Check sheet for the modelled part. Datum: model origin and axes. Units: mm. Face numbers are marked on the shaded views. A direction names the side the tool comes from. Coordinates: 2 decimals unless noted, no trailing zeros. Write each loop counter-clockwise with the first axis right and the second up, starting at its lowest first coordinate (ties: lowest second). Pieces come first, ordered by that corner, then holes. Notation, with made-up numbers: (12.25, 49.25) - (28.25, 49.25) arc R27 cw to (28.25, 70.25) - close; hole circle Ø4 at (-0.5, 62). An arc over 180 degrees is marked (long way). Write each question's results on one line, items separated by ' | '.
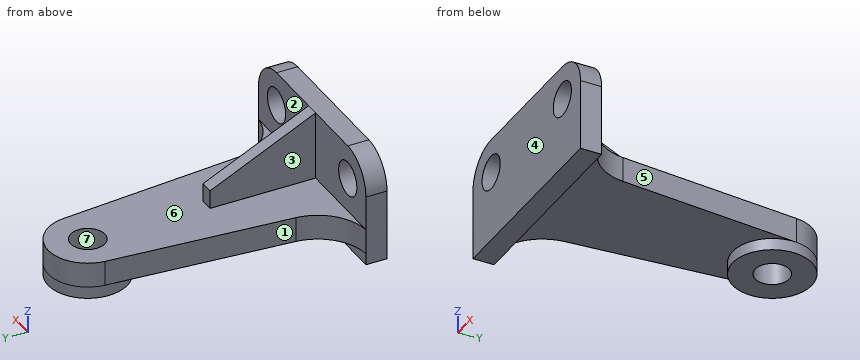
from build123d import *

# Parameters (mm, degrees)
EXTRUDE_1_DEPTH     = 8
SKETCH_2_R          = 6.5
CUT_EXTRUDE_1_DEPTH = 8
EXTRUDE_2_DEPTH     = 9.5
SKETCH_4_R          = 15
EXTRUDE_3_DEPTH     = 4.5
SKETCH_5_R          = 6.5
CUT_EXTRUDE_2_DEPTH = 41
EXTRUDE_4_DEPTH     = 2.5


with BuildPart() as part:
    # 스케치1 → 보스-돌출1 (new body)
    with BuildSketch(Plane(origin=(0, 0, 0), x_dir=(1, 0, 0), z_dir=(0, 1, 0))):
        with BuildLine():
            Line((-38.5, 40), (38.5, 40))
            Line((38.5, 40), (38.5, 13))
            ThreePointArc((38.5, 13), (34.692388155, 3.807611845), (25.5, 0))
            Line((25.5, 0), (-25.5, 0))
            ThreePointArc((-25.5, 0), (-34.692388155, 3.807611845), (-38.5, 13))
            Line((-38.5, 13), (-38.5, 40))
        make_face()
    extrude(amount=EXTRUDE_1_DEPTH)

    # 스케치2 → 컷-돌출1 (cut)
    with BuildSketch(Plane(origin=(0, 8, 0), x_dir=(1, 0, 0), z_dir=(0, 1, 0))):
        with Locations((-25.5, 13)):
            Circle(SKETCH_2_R)
        with Locations((25.5, 13)):
            Circle(SKETCH_2_R)
    extrude(amount=-CUT_EXTRUDE_1_DEPTH, mode=Mode.SUBTRACT)

    # 스케치3 → 보스-돌출2 (add)
    with BuildSketch(Plane(origin=(0, 0, -26), x_dir=(-1, 0, 0), z_dir=(0, 0, -1))):
        with BuildLine():
            Line((-38.5, 0), (-38.5, 8))
            ThreePointArc((-38.5, 8), (-26.561663341, 13.425258865), (-20.981002143, 25.291746827))
            Line((-20.981002143, 25.291746827), (-14.942920471, 94.307336141))
            ThreePointArc((-14.942920471, 94.307336141), (0, 108), (14.942920471, 94.307336141))
            Line((14.942920471, 94.307336141), (20.981002143, 25.291746827))
            ThreePointArc((20.981002143, 25.291746827), (26.561663341, 13.425258865), (38.5, 8))
            Line((38.5, 8), (38.5, 0))
            Line((38.5, 0), (-38.5, 0))
        make_face()
    extrude(amount=EXTRUDE_2_DEPTH)

    # 스케치4 → 보스-돌출3 (add)
    with BuildSketch(Plane(origin=(0, 0, -35.5), x_dir=(-1, 0, 0), z_dir=(0, 0, -1))):
        with Locations((0, 93)):
            Circle(SKETCH_4_R)
    extrude(amount=EXTRUDE_3_DEPTH)

    # 스케치5 → 컷-돌출2 (cut, through all)
    with BuildSketch(Plane(origin=(0, 0, -40), x_dir=(-1, 0, 0), z_dir=(0, 0, -1))):
        with Locations((0, 93)):
            Circle(SKETCH_5_R)
    extrude(amount=-CUT_EXTRUDE_2_DEPTH, mode=Mode.SUBTRACT)

    # 스케치7 → 보스-돌출4 (add, symmetric)
    with BuildSketch(Plane(origin=(0, 0, 0), x_dir=(0, 0, -1), z_dir=(1, 0, 0))):
        Polygon((0, 8), (35.5, 8), (35.5, 48), (19, 48), align=None)
    extrude(amount=EXTRUDE_4_DEPTH, both=True)


solid = part.part
1. Material ranges on L1, parallel to X at y = 3.25, z = -13; L2, parallel to Y at x = 0, z = -35.25; L3, parallel to Z at x = 25, y = 3, recorded low to high. Write a range as [from, to].
Values follow:
L1: x = [-38.5, -32], [-19, 19], [32, 38.5] | L2: y = [0, 86.5], [99.5, 108] | L3: z = [-40, -19.48], [-6.52, 0]
2. Sectioned sample at A-A (z = -28). Record the cut outline in (x, y), then the cut area to 3 significant figures.
Values follow:
outline: (-38.5, 0) - (38.5, 0) - (38.5, 8) arc R19 cw to (20.98, 25.29) - (14.94, 94.31) arc R15 ccw to (-14.94, 94.31) - (-20.98, 25.29) arc R19 cw to (-38.5, 8) - close; hole circle Ø13 at (0, 93) | area: 4,150 mm^2
3. Sectioned sample at C-C (z = -9). Record the cut outline in (x, y).
Values follow:
outline: (-37.87, 0) - (-30.62, 0) - (-30.62, 8) - (-37.87, 8) - close; (-20.38, 0) - (20.38, 0) - (20.38, 8) - (2.5, 8) - (2.5, 26.95) - (-2.5, 26.95) - (-2.5, 8) - (-20.38, 8) - close; (30.62, 0) - (37.87, 0) - (37.87, 8) - (30.62, 8) - close
4. Go/stop test with flat-tipped pins: pin 1 (1 mm diameter, centred on y = 42, z = -19.5, fed in from -X); pin 2 (21 mm diameter, centred on x = -25.5, z = -13, fed in from -Y); pin 3 (6 mm diameter, centred on x = -9.5, y = 46, fed in from +Z); pin 4 (23 mm diameter, centred on x = 15, y = 61.5, fed in from -Z). Record where each tip stops, or that it passes through.
Values follow:
pin 1: stops at x = -2.5 | pin 2: stops at y = 0 | pin 3: stops at z = -26 | pin 4: stops at z = -35.5
5. Access from +Z, -Z, +X, -X, +Y, -Y to the whole of each face (thin tool, end or side, straight path). Record for the marked faces 1, 2 and 3.
Values follow:
face 1: +Z, -Z, -X, +Y | face 2: +Z, +X, +Y | face 3: +Z, -X, +Y
6. Draft check along Y on the marked faces 4, 5, 6 and 7. Enter one of: pulls with the +Y half, pulls with the -Y half, needs draft (parallel to the pull), parting line crosses it, or undercut.
Values follow:
face 4: pulls with the -Y half | face 5: pulls with the +Y half | face 6: needs draft | face 7: undercut
7. Sectioned sample at B-B (x = -29). Record the cut outline in (y, z), then the cut area to 3 significant figures.
Values follow:
outline: (0, -40) - (8, -40) - (8, -35.5) - (11.39, -35.5) - (11.39, -26) - (8, -26) - (8, -18.48) - (0, -18.48) - close; (0, -7.52) - (8, -7.52) - (8, -0.48) - (0, -0.48) - close | area: 261 mm^2
8. Sectioned sample at D-D (y = 93). Record the cut outline in (x, z), then the cut area to 3 significant figures.
Values follow:
outline: (-15.06, -35.5) - (-15, -35.5) - (-15, -40) - (-6.5, -40) - (-6.5, -26) - (-15.06, -26) - close; (6.5, -40) - (15, -40) - (15, -35.5) - (15.06, -35.5) - (15.06, -26) - (6.5, -26) - close | area: 239 mm^2
